The model under review builds one solid part; all positions refer to its coordinate system, in mm. Round coordinates to 2 decimals unless told otherwise and drop trailing zeros. Loops run counter-clockwise (first coordinate to the right, second up) from the corner with the lowest first, then second, coordinate; pieces in that order, holes last. Notation, with made-up numbers: (5, 52.5) -> (59, 52.5) arc R30 cw to (59, 88.5) -> close; hole circle Ø1 at (-32.5, -37). An arc over 180 degrees is marked (long way). Write each question's results on one line, items separated by ' | '. Start each with the question number.
Item 1: Clearance check with flat-ended pins moving along their axes: pin 1 Ø3 at (y, z) = (12.5, 39.5) entering from +X; pin 2 Ø3 at (y, z) = (15, -183) entering from +X; pin 3 Ø4 at (y, z) = (15, 31.5) entering from +X; pin 4 Ø10 at (y, z) = (18.5, -141.5) entering from +X. State where each tip first meets the part, or that it passes through.
Item 2: We need section A-A (x = 8). Give the boundary of the cut face in (y, z).
Item 3: For L1, parallel to Y at x = -62.75, z = -167; L2, parallel to Z at x = 40, y = 22; L3, parallel to Z at x = 34, y = 10, list the stretches that pass through material, from the lowest coordinate up. Write a range as from..to.
Item 4: We need section B-B (z = -72.5). Give the boundary of the cut face in (x, y), and give its area (3 significant figures).
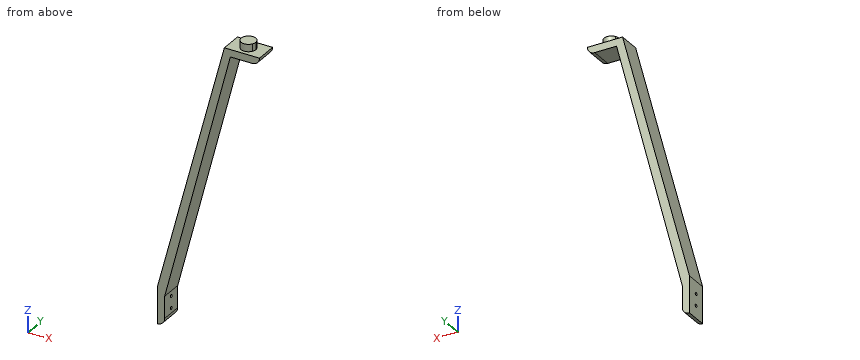
from build123d import *

# Parameters (mm, degrees)
ESQUISSE1_W             = 140
ESQUISSE1_H             = 400
BOSS_EXTRU_1_DEPTH      = 30
ENL_V_MAT_EXTRU_2_DEPTH = 30
ESQUISSE3_R             = 2
ENL_V_MAT_EXTRU_3_DEPTH = 246.967477525
BOSS_EXTRU_3_DEPTH      = 10
CONG_1_R                = 10
CONG_2_R                = 10


with BuildPart() as part:
    # Esquisse1 → Boss.-Extru.1 (new body)
    with BuildSketch(Plane(origin=(0, 0, 0), x_dir=(1, 0, 0), z_dir=(0, 1, 0))):
        Rectangle(ESQUISSE1_W, ESQUISSE1_H)
    extrude(amount=BOSS_EXTRU_1_DEPTH)

    # Esquisse2 → Enlèv. mat.-Extru.2 (cut)
    with BuildSketch(Plane(origin=(0, 30, 0), x_dir=(1, 0, 0), z_dir=(0, 1, 0))):
        Polygon((21.786415215, -200), (-70, 150), (-70, -200), align=None)
        Polygon((70, 200), (-60, 200), (-60, 160), (30, -190), (70, -190), align=None)
    extrude(amount=-ENL_V_MAT_EXTRU_2_DEPTH, mode=Mode.SUBTRACT)

    # Esquisse3 → Enlèv. mat.-Extru.3 (cut, through all)
    with BuildSketch(Plane.ZY.offset(70)):
        with Locations((-183, 15)):
            Circle(ESQUISSE3_R)
        with Locations((-167, 15)):
            Circle(ESQUISSE3_R)
    extrude(amount=-ENL_V_MAT_EXTRU_3_DEPTH, mode=Mode.SUBTRACT)

    # Esquisse4 → Boss.-Extru.3 (add)
    with BuildSketch(Plane.XY.offset(200)):
        with BuildLine():
            ThreePointArc((55.893207608, 15), (48.640450238, 24.615230519), (37.402676021, 20.283074236))
            Line((37.402676021, 20.283074236), (54.383739194, 9.716925764))
            ThreePointArc((54.383739194, 9.716925764), (55.508438127, 12.25275737), (55.893207608, 15))
        make_face()
        with BuildLine():
            Line((54.383739194, 9.716925764), (37.402676021, 20.283074236))
            ThreePointArc((37.402676021, 20.283074236), (40.610133372, 6.509468414), (54.383739194, 9.716925764))
        make_face()
    extrude(amount=BOSS_EXTRU_3_DEPTH)

    # Congé1
    cong_1_edges = [part.edges().sort_by_distance(p)[0] for p in [
        (-60, 15, -200),
    ]]
    fillet(cong_1_edges, radius=CONG_1_R - 0.0001)  # a hair under: the kernel refuses the full size

    # Congé2
    cong_2_edges = [part.edges().sort_by_distance(p)[0] for p in [
        (70, 15, 190),
    ]]
    fillet(cong_2_edges, radius=CONG_2_R - 0.0001)  # a hair under: the kernel refuses the full size


solid = part.part
Here are the results:
1) pin 1: stops at x = -8.31 | pin 2: passes through | pin 3: stops at x = -10.24 | pin 4: stops at x = -53.96
2) outline: (0, 104.44) -> (30, 104.44) -> (30, 147.43) -> (0, 147.43) -> close
3) L1: y = 0..13, 17..30 | L2: z = 190..210 | L3: z = 190..200
4) outline: (-49.68, 0) -> (-37.5, 0) -> (-37.5, 30) -> (-49.68, 30) -> close | area: 365 mm2
